Could you check a few things on this model? Use its own coordinates, in mm. A direction names the side the tool comes from. Coordinates: 2 decimals unless noted, no trailing zeros. Order: outer loops, then holes, each group sorted by start corner. A loop starts at its lowest first (then second) coordinate and runs counter-clockwise, first axis right, second up. Notation, with made-up numbers: (51.25, -24.5) -> (89.25, -24.5) arc R30 cw to (89.25, 7.5) -> close; hole circle Ø10 at (32, -18.5). An arc over 180 degrees is marked (long way). Put each result on its own line as item: value. Start each with the question number.
Q1. Will these pins go through, and if not, where does the flat tip stop? pin 1 (2.5 mm diameter, centred on y = 3.5, z = -24.5, fed in from +X); pin 2 (10 mm diameter, centred on x = 17, y = 16, fed in from -Z); pin 3 (8 mm diameter, centred on y = 5, z = -22.5, fed in from -X).
Q2. For faces 1 (the face through (12.5, 16.5, -23.6)), 2 (the face through (19.62, 11.48, -8.76)), 3 (the face through (-7.6, 8, -22.3)), 4 (the face through (7.578, 12.479, -20.716)), 5 (the face through (0, 16, -17)), which set-ups out of +Z, -Z, +X, -X, +Y, -Y let a thin tool reach every point of the face, with its end or its side?
Q3. If we section it at D-D (z = -14.25): Please give me the cut outline in (x, y).
Q4. We'd pull the mould along Y, two halves only. Please class faces 6 (the face through (0, 15, -12)), 7 (the face through (-19.426, 7.395, -16.721)), 8 (the face through (-7.62, 3.48, -20.74)): +Y half, -Y half, draft (parallel to the pull), parting line (faces both ways), or undercut.
Q5. Please list where these lines run through material, in increasing order: line 1 along Y through (x, z) = (-20, -6.5); line 2 along Y through (x, z) = (-3.5, -22.25); line 3 along Z through (x, y) = (6, 14.95).
Q6. If we section it at B-B (z = -3.25): Please give me the cut outline in (x, y).
Q7. If we section it at A-A (x = 6.5): Count the separate pieces of the cut face and the enclosed holes in it, and give its area (3 significant figures).
Q8. If we section it at C-C (y = 12): Please give me the cut outline in (x, z).
from build123d import *

# Parameters (mm, degrees)
SKETCH1_R           = 2
BOSS_EXTRUDE1_DEPTH = 15
SKETCH2_R           = 2
BOSS_EXTRUDE2_DEPTH = 3
SKETCH5_W           = 6.4
SKETCH5_H           = 3
CUT_EXTRUDE1_DEPTH  = 6.4
CUT_EXTRUDE2_DEPTH  = 3
CUT_EXTRUDE3_DEPTH  = 3
SKETCH8_W           = 6.4
SKETCH8_H           = 3
CUT_EXTRUDE4_DEPTH  = 6
CUT_EXTRUDE5_DEPTH  = 3
CUT_EXTRUDE6_DEPTH  = 3


with BuildPart() as part:
    # Sketch1 → Boss-Extrude1 (new body)
    with BuildSketch(Plane(origin=(0, 0, 0), x_dir=(1, 0, 0), z_dir=(0, 1, 0))):
        with BuildLine():
            Line((-18.062870566, 0), (18.062870566, 0))
            ThreePointArc((18.062870566, 0), (22.119081492, 2.076448577), (22.806287057, 6.58113883))
            Line((22.806287057, 6.58113883), (16.13962039, 26.58113883))
            ThreePointArc((16.13962039, 26.58113883), (14.319755323, 29.056210926), (11.3962039, 30))
            Line((11.3962039, 30), (-11.3962039, 30))
            ThreePointArc((-11.3962039, 30), (-14.319755323, 29.056210926), (-16.13962039, 26.58113883))
            Line((-16.13962039, 26.58113883), (-22.806287057, 6.58113883))
            ThreePointArc((-22.806287057, 6.58113883), (-22.119081492, 2.076448577), (-18.062870566, 0))
        make_face()
        with Locations((-18, 6)):
            Circle(SKETCH1_R, mode=Mode.SUBTRACT)
        with Locations((18, 6)):
            Circle(SKETCH1_R, mode=Mode.SUBTRACT)
        with Locations((6, 23.5)):
            Circle(SKETCH1_R, mode=Mode.SUBTRACT)
        with Locations((-6, 23.5)):
            Circle(SKETCH1_R, mode=Mode.SUBTRACT)
    extrude(amount=BOSS_EXTRUDE1_DEPTH)

    # Sketch2 → Boss-Extrude2 (add)
    with BuildSketch(Plane(origin=(0, 15, 0), x_dir=(1, 0, 0), z_dir=(0, 1, 0))):
        with BuildLine():
            Line((-6, 30), (6, 30))
            ThreePointArc((6, 30), (12.5, 23.5), (6, 17))
            Line((6, 17), (-6, 17))
            ThreePointArc((-6, 17), (-12.5, 23.5), (-6, 30))
        make_face()
        with Locations((-6, 23.5)):
            Circle(SKETCH2_R, mode=Mode.SUBTRACT)
        with Locations((6, 23.5)):
            Circle(SKETCH2_R, mode=Mode.SUBTRACT)
    extrude(amount=BOSS_EXTRUDE2_DEPTH)

    # Sketch5 → Cut-Extrude1 (cut)
    with BuildSketch(Plane(origin=(0, 0, -30), x_dir=(-1, 0, 0), z_dir=(0, 0, -1))):
        with Locations((6, 12.5)):
            Rectangle(SKETCH5_W, SKETCH5_H)
        with Locations((-6, 12.5)):
            Rectangle(SKETCH5_W, SKETCH5_H)
        with Locations((-6, 3.5)):
            Rectangle(SKETCH5_W, SKETCH5_H)
        with Locations((6, 3.5)):
            Rectangle(SKETCH5_W, SKETCH5_H)
    extrude(amount=-CUT_EXTRUDE1_DEPTH, mode=Mode.SUBTRACT)

    # Sketch6 → Cut-Extrude2 (cut)
    with BuildSketch(Plane(origin=(0, 11, 0), x_dir=(1, 0, 0), z_dir=(0, 1, 0))):
        Polygon((9.2, 25.347520861), (6, 27.195041723), (2.8, 25.347520861), (2.8, 21.652479139), (6, 19.804958277), (9.2, 21.652479139), align=None)
        Polygon((-2.8, 25.347520861), (-6, 27.195041723), (-9.2, 25.347520861), (-9.2, 21.652479139), (-6, 19.804958277), (-2.8, 21.652479139), align=None)
    extrude(amount=CUT_EXTRUDE2_DEPTH, mode=Mode.SUBTRACT)

    # Sketch7 → Cut-Extrude3 (cut)
    with BuildSketch(Plane(origin=(0, 2, 0), x_dir=(1, 0, 0), z_dir=(0, 1, 0))):
        Polygon((9.2, 25.347520861), (6, 27.195041723), (2.8, 25.347520861), (2.8, 21.652479139), (6, 19.804958277), (9.2, 21.652479139), align=None)
        Polygon((-6, 19.804958277), (-2.8, 21.652479139), (-2.8, 25.347520861), (-6, 27.195041723), (-9.2, 25.347520861), (-9.2, 21.652479139), align=None)
    extrude(amount=CUT_EXTRUDE3_DEPTH, mode=Mode.SUBTRACT)

    # Sketch8 → Cut-Extrude4 (cut)
    with BuildSketch(Plane.XY):
        with Locations((18, 11.5)):
            Rectangle(SKETCH8_W, SKETCH8_H)
        with Locations((-18, 11.5)):
            Rectangle(SKETCH8_W, SKETCH8_H)
        with Locations((-18, 3.5)):
            Rectangle(SKETCH8_W, SKETCH8_H)
        with Locations((18, 3.5)):
            Rectangle(SKETCH8_W, SKETCH8_H)
    extrude(amount=-CUT_EXTRUDE4_DEPTH, mode=Mode.SUBTRACT)

    # Sketch9 → Cut-Extrude5 (cut)
    with BuildSketch(Plane(origin=(0, 10, 0), x_dir=(1, 0, 0), z_dir=(0, 1, 0))):
        Polygon((21.2, 4.152479139), (21.2, 7.847520861), (18, 9.695041723), (14.8, 7.847520861), (14.8, 4.152479139), (18, 2.304958277), align=None)
        Polygon((-14.8, 4.152479139), (-14.8, 7.847520861), (-18, 9.695041723), (-21.2, 7.847520861), (-21.2, 4.152479139), (-18, 2.304958277), align=None)
    extrude(amount=CUT_EXTRUDE5_DEPTH, mode=Mode.SUBTRACT)

    # Sketch10 → Cut-Extrude6 (cut)
    with BuildSketch(Plane(origin=(0, 2, 0), x_dir=(1, 0, 0), z_dir=(0, 1, 0))):
        Polygon((21.2, 4.152479139), (21.2, 7.847520861), (18, 9.695041723), (14.8, 7.847520861), (14.8, 4.152479139), (18, 2.304958277), align=None)
        Polygon((-21.2, 4.152479139), (-18, 2.304958277), (-14.8, 4.152479139), (-14.8, 7.847520861), (-18, 9.695041723), (-21.2, 7.847520861), align=None)
    extrude(amount=CUT_EXTRUDE6_DEPTH, mode=Mode.SUBTRACT)


solid = part.part
The answers:
1. pin 1: x = 17.25
1. pin 2: z = -29.95
1. pin 3: x = -18.83
2. face 1: +X, +Y
2. face 2: +Z
2. face 3: +Y, -Y
2. face 4: -Z
2. face 5: +Z, +X, -X, +Y
3. outline: (-20.25, 0) -> (20.25, 0) -> (20.25, 15) -> (-20.25, 15) -> close
4. face 6: +Y half
4. face 7: draft
4. face 8: undercut
5. line 1: 0 to 2, 5 to 10, 13 to 15
5. line 2: 0 to 2, 5 to 11, 14 to 18
5. line 3: -30 to -25.5, -21.5 to 0
6. outline: (-22.75, 0) -> (22.75, 0) -> (22.75, 15) -> (-22.75, 15) -> close; hole (-21.2, 2) -> (-14.8, 2) -> (-14.8, 5) -> (-21.2, 5) -> close; hole (-21.2, 10) -> (-14.8, 10) -> (-14.8, 13) -> (-21.2, 13) -> close; hole (14.8, 2) -> (21.2, 2) -> (21.2, 5) -> (14.8, 5) -> close; hole (14.8, 10) -> (21.2, 10) -> (21.2, 13) -> (14.8, 13) -> close
7. separate pieces: 4
7. enclosed holes: 0
7. area: 383 mm^2
8. outline: (-22.81, -6.58) -> (-16.14, -26.58) arc R5 ccw to (-11.4, -30) -> (-9.2, -30) -> (-9.2, -21.65) -> (-6, -19.8) -> (-2.8, -21.65) -> (-2.8, -30) -> (2.8, -30) -> (2.8, -21.65) -> (6, -19.8) -> (9.2, -21.65) -> (9.2, -30) -> (11.4, -30) arc R5 ccw to (16.14, -26.58) -> (22.81, -6.58) arc R5 ccw to (21.2, -1.11) -> (21.2, -7.85) -> (18, -9.7) -> (14.8, -7.85) -> (14.8, 0) -> (-14.8, 0) -> (-14.8, -7.85) -> (-18, -9.7) -> (-21.2, -7.85) -> (-21.2, -1.11) arc R5 ccw to start
